from build123d import *

# Parameters (mm, degrees)
SKETCH1_R           = 6.5
BOSS_EXTRUDE1_DEPTH = 67.5
CUT_EXTRUDE1_START  = 6.5
CUT_EXTRUDE1_DEPTH  = 1.5


with BuildPart() as part:
    # Sketch1 → Boss-Extrude1 (new, symmetric)
    with BuildSketch(Plane.XY):
        Circle(SKETCH1_R)
    extrude(amount=BOSS_EXTRUDE1_DEPTH, both=True)

    # Sketch2 → Cut-Extrude1 (cut)
    with BuildSketch(Plane(origin=(0, 0, 0), x_dir=(0, 0, -1), z_dir=(1, 0, 0)).offset(CUT_EXTRUDE1_START)):
        with BuildLine():
            Line((-26.5, 1.5), (8.5, 1.5))
            ThreePointArc((8.5, 1.5), (10, 0), (8.5, -1.5))
            Line((8.5, -1.5), (-26.5, -1.5))
            ThreePointArc((-26.5, -1.5), (-28, 0), (-26.5, 1.5))
        make_face()
    extrude(amount=-CUT_EXTRUDE1_DEPTH, mode=Mode.SUBTRACT)


solid = part.part
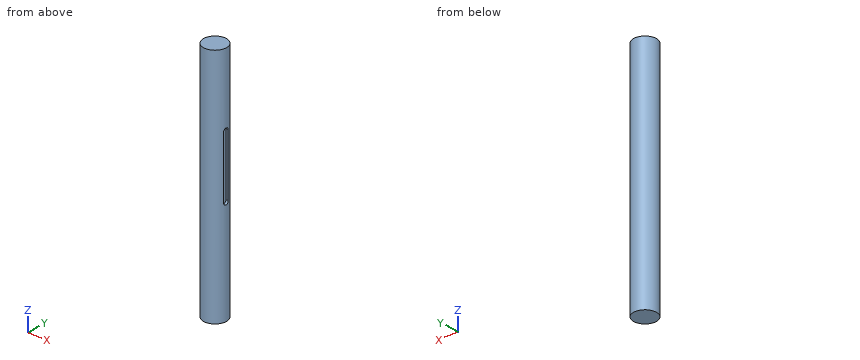
Build history of the part. All positions in model axes, mm. Coordinates: 2 decimals unless noted, no trailing zeros. Order: outer loops, then holes, each group sorted by start corner. A loop starts at its lowest first (then second) coordinate and runs counter-clockwise, first axis right, second up. Notation, with made-up numbers: (8, -7.5) -> (55, -7.5) arc R32 ccw to (55, 18.5) -> close; hole circle Ø3 at (71.25, -25.5). An arc over 180 degrees is marked (long way). One line per item, written item: value.
(1) Drop flat-ended pins along their axis: pin 1 Ø1.5 at (y, z) = (0.5, 9) entering from +X; pin 2 Ø0.7 at (x, z) = (5.5, 11) entering from +Y; pin 3 Ø4 at (x, z) = (-2.5, -36) entering from -Y. Give the stop position or say it passes through.
Checked values:
pin 1: x = 5
pin 2: y = 3.97
pin 3: y = -6.48
(2) Probe line 1 (X direction, y = -0.25, z = 6); line 2 (Y direction, x = 5, z = -14); line 3 (Y direction, x = -4.5, z = 11). List the from-to ranges inside material, lowest first. Write a range as [from, to].
Checked values:
line 1: [-6.5, 5]
line 2: [-4.15, 4.15]
line 3: [-4.69, 4.69]
(3) Slice it at A-A, the plane y = 0. List the corners of the cut face in (x, z).
Checked values:
outline: (-6.5, -67.5) -> (6.5, -67.5) -> (6.5, -10) -> (5, -10) -> (5, 28) -> (6.5, 28) -> (6.5, 67.5) -> (-6.5, 67.5) -> close
(4) Slice it at C-C, the plane x = -2.75. List the corners of the cut face in (y, z), plus the area to 3 significant figures.
Checked values:
outline: (-5.89, -67.5) -> (5.89, -67.5) -> (5.89, 67.5) -> (-5.89, 67.5) -> close
area: 1,590 mm2
(5) Slice it at B-B, the plane z = -12.5. List the corners of the cut face in (x, y), plus the area to 3 significant figures.
Checked values:
outline: circle Ø13 at (0, 0)
area: 133 mm2
(6) Slice it at D-D, the plane x = 3.5. List the corners of the cut face in (y, z), plus the area to 3 significant figures.
Checked values:
outline: (-5.48, -67.5) -> (5.48, -67.5) -> (5.48, 67.5) -> (-5.48, 67.5) -> close
area: 1,480 mm2
